CAD build for the part. Positions are in the model's coordinates, mm. A direction names the side the tool comes from. Give positions to 0.01 mm unless a question says otherwise; leave off trailing zeros. Order: outer loops, then holes, each group sorted by start corner. A loop starts at its lowest first (then second) coordinate and runs counter-clockwise, first axis right, second up.
Item 1: Wall check: L1, parallel to X at y = -5.25, z = -1.2; L2, parallel to Y at x = 15.25, z = -0.85; L3, parallel to Y at x = 32.25, z = 0.6. Give the ranges that are in metal, low to high.
Item 2: Flat gauge pins, fed straight in: P1, Ø4, axis at x = 31.46, y = -10.9, coming from the +Z side; P2, Ø2, axis at y = -8.5, z = -2, coming from the +X side; P3, Ø1.2, axis at x = 21.5, z = -1.5, coming from the -Y side; P4, Ø2.5, axis at x = 16, y = -10, coming from the -Z side. Where does each tip first touch, or does it go through?
Item 3: Two-plate mould, pull along X, no slides. Class faces 4 (the flat face through (13.37, -9.09, 0.49)), 5 (the conical face through (34.4, -13.8, 0.6)), 6 (the conical face through (6.94, -13.798, 0.618)), 7 (the flat face through (20, -13.101, -1)): released by +X, released by -X, zero draft, split by the parting line, or undercut.
Item 4: Band-saw the part on B-B on y = -8.75. Give the cut face in (x, z).
Item 5: Which spindle directions (+Z, -Z, +X, -X, +Y, -Y) get a long thin tool onto all of the face, cutting with end or side? Do faces 1 (the flat face through (7.664, -8, -1)), 2 (the flat face through (24.17, -9.09, 0.49)), 3 (the flat face through (8.9, -4.5, 0)). Say none if no direction does.
Item 6: Band-saw the part on D-D on y = -10.5. Count the separate pieces of the cut face and the enclosed holes in it, plus the area to 3 significant figures.
Item 7: Band-saw the part on A-A on z = -0.9. Give the cut face in (x, y), plus the area to 3 significant figures.
Item 8: Band-saw the part on C-C on x = 25.5. Give the cut face in (y, z), plus the area to 3 significant figures.
```python
from build123d import *

# Parameters (mm, degrees)
SKETCH_1_W          = 26
SKETCH_1_H          = 9.8
SKETCH_1_W_2        = 24
SKETCH_1_H_2        = 7.8
EXTRUDE_1_DEPTH     = 2.5
EXTRUDE_2_DEPTH     = 1
EXTRUDE_2_TAPER     = 25
CUT_EXTRUDE_1_REACH = 3
SKETCH_3_R          = 1.2


with BuildPart() as part:
    # 草图1 → 凸台-拉伸1 (new body)
    with BuildSketch(Plane.XY):
        with Locations((20.66383505, -8.200793938)):
            Rectangle(SKETCH_1_W, SKETCH_1_H)
        with Locations((20.66383505, -8.200793938)):
            Rectangle(SKETCH_1_W_2, SKETCH_1_H_2, mode=Mode.SUBTRACT)
    extrude(amount=-EXTRUDE_1_DEPTH)

    # 草图2 → 凸台-拉伸2 (add)
    with BuildSketch(Plane.XY):
        with BuildLine():
            Line((35.16383505, -12.600793938), (35.16383505, -3.800793938))
            ThreePointArc((35.16383505, -3.800793938), (34.578048612, -2.386580376), (33.16383505, -1.800793938))
            Line((33.16383505, -1.800793938), (8.16383505, -1.800793938))
            ThreePointArc((8.16383505, -1.800793938), (6.749621488, -2.386580376), (6.16383505, -3.800793938))
            Line((6.16383505, -3.800793938), (6.16383505, -12.600793938))
            ThreePointArc((6.16383505, -12.600793938), (6.749621488, -14.015007501), (8.16383505, -14.600793938))
            Line((8.16383505, -14.600793938), (33.16383505, -14.600793938))
            ThreePointArc((33.16383505, -14.600793938), (34.578048612, -14.015007501), (35.16383505, -12.600793938))
        make_face()
    extrude(amount=EXTRUDE_2_DEPTH, taper=EXTRUDE_2_TAPER)

    # 草图3 → 切除-拉伸1 (cut, up to next)
    with BuildSketch(Plane(origin=(0, 0, 0), x_dir=(-1, 0, 0), z_dir=(0, 0, -1)), mode=Mode.PRIVATE) as cut_extrude_1_sk1:
        with Locations((-31.46383505, -10.900793938)):
            Circle(SKETCH_3_R)
    cut_extrude_1_tool1 = extrude(cut_extrude_1_sk1.sketch, amount=-CUT_EXTRUDE_1_REACH, mode=Mode.PRIVATE) & part.part
    add(cut_extrude_1_tool1.solids().sort_by_distance((31.463835, -10.900794, 0))[0], mode=Mode.SUBTRACT)
    # 草图3 → 切除-拉伸1 (cut, up to next)
    with BuildSketch(Plane(origin=(0, 0, 0), x_dir=(-1, 0, 0), z_dir=(0, 0, -1)), mode=Mode.PRIVATE) as cut_extrude_1_sk2:
        with Locations((-9.86383505, -5.500793938)):
            Circle(SKETCH_3_R)
    cut_extrude_1_tool2 = extrude(cut_extrude_1_sk2.sketch, amount=-CUT_EXTRUDE_1_REACH, mode=Mode.PRIVATE) & part.part
    add(cut_extrude_1_tool2.solids().sort_by_distance((9.863835, -5.500794, 0))[0], mode=Mode.SUBTRACT)
    # 草图3 → 切除-拉伸1 (cut, up to next)
    with BuildSketch(Plane(origin=(0, 0, 0), x_dir=(-1, 0, 0), z_dir=(0, 0, -1)), mode=Mode.PRIVATE) as cut_extrude_1_sk3:
        with BuildLine():
            Line((-30.615306913, -4.652265801), (-25.215306913, -10.052265801))
            ThreePointArc((-25.215306913, -10.052265801), (-25.215306913, -11.749322076), (-26.912363188, -11.749322076))
            Line((-26.912363188, -11.749322076), (-32.312363188, -6.349322076))
            ThreePointArc((-32.312363188, -6.349322076), (-32.312363188, -4.652265801), (-30.615306913, -4.652265801))
        make_face()
    cut_extrude_1_tool3 = extrude(cut_extrude_1_sk3.sketch, amount=-CUT_EXTRUDE_1_REACH, mode=Mode.PRIVATE) & part.part
    add(cut_extrude_1_tool3.solids().sort_by_distance((28.763835, -8.200794, 0))[0], mode=Mode.SUBTRACT)
    # 草图3 → 切除-拉伸1 (cut, up to next)
    with BuildSketch(Plane(origin=(0, 0, 0), x_dir=(-1, 0, 0), z_dir=(0, 0, -1)), mode=Mode.PRIVATE) as cut_extrude_1_sk4:
        with BuildLine():
            Line((-25.215306913, -4.652265801), (-19.815306913, -10.052265801))
            ThreePointArc((-19.815306913, -10.052265801), (-19.815306913, -11.749322076), (-21.512363188, -11.749322076))
            Line((-21.512363188, -11.749322076), (-26.912363188, -6.349322076))
            ThreePointArc((-26.912363188, -6.349322076), (-26.912363188, -4.652265801), (-25.215306913, -4.652265801))
        make_face()
    cut_extrude_1_tool4 = extrude(cut_extrude_1_sk4.sketch, amount=-CUT_EXTRUDE_1_REACH, mode=Mode.PRIVATE) & part.part
    add(cut_extrude_1_tool4.solids().sort_by_distance((23.363835, -8.200794, 0))[0], mode=Mode.SUBTRACT)
    # 草图3 → 切除-拉伸1 (cut, up to next)
    with BuildSketch(Plane(origin=(0, 0, 0), x_dir=(-1, 0, 0), z_dir=(0, 0, -1)), mode=Mode.PRIVATE) as cut_extrude_1_sk5:
        with BuildLine():
            Line((-19.815306913, -4.652265801), (-14.415306913, -10.052265801))
            ThreePointArc((-14.415306913, -10.052265801), (-14.415306913, -11.749322076), (-16.112363188, -11.749322076))
            Line((-16.112363188, -11.749322076), (-21.512363188, -6.349322076))
            ThreePointArc((-21.512363188, -6.349322076), (-21.512363188, -4.652265801), (-19.815306913, -4.652265801))
        make_face()
    cut_extrude_1_tool5 = extrude(cut_extrude_1_sk5.sketch, amount=-CUT_EXTRUDE_1_REACH, mode=Mode.PRIVATE) & part.part
    add(cut_extrude_1_tool5.solids().sort_by_distance((17.963835, -8.200794, 0))[0], mode=Mode.SUBTRACT)
    # 草图3 → 切除-拉伸1 (cut, up to next)
    with BuildSketch(Plane(origin=(0, 0, 0), x_dir=(-1, 0, 0), z_dir=(0, 0, -1)), mode=Mode.PRIVATE) as cut_extrude_1_sk6:
        with BuildLine():
            Line((-14.415306913, -4.652265801), (-9.015306913, -10.052265801))
            ThreePointArc((-9.015306913, -10.052265801), (-9.015306913, -11.749322076), (-10.712363188, -11.749322076))
            Line((-10.712363188, -11.749322076), (-16.112363188, -6.349322076))
            ThreePointArc((-16.112363188, -6.349322076), (-16.112363188, -4.652265801), (-14.415306913, -4.652265801))
        make_face()
    cut_extrude_1_tool6 = extrude(cut_extrude_1_sk6.sketch, amount=-CUT_EXTRUDE_1_REACH, mode=Mode.PRIVATE) & part.part
    add(cut_extrude_1_tool6.solids().sort_by_distance((12.563835, -8.200794, 0))[0], mode=Mode.SUBTRACT)


solid = part.part
```
The answers:
1. L1: x = 7.66 to 8.66, 32.66 to 33.66
1. L2: y = -13.1 to -12.1, -4.3 to -3.3
1. L3: y = -14.32 to -11.81, -9.99 to -6.41, -4.59 to -2.08
2. P1: stops at z = 1
2. P2: stops at x = 33.66
2. P3: stops at y = -13.1
2. P4: stops at z = 0
3. face 4: undercut
3. face 5: released by +X
3. face 6: released by -X
3. face 7: zero draft
4. outline: (6.16, 0) - (7.66, 0) - (7.66, -2.5) - (8.66, -2.5) - (8.66, 0) - (10.32, 0) - (10.32, 1) - (6.63, 1) - close; (13.71, 0) - (15.72, 0) - (15.72, 1) - (13.71, 1) - close; (19.11, 0) - (21.12, 0) - (21.12, 1) - (19.11, 1) - close; (24.51, 0) - (26.52, 0) - (26.52, 1) - (24.51, 1) - close; (29.91, 0) - (32.66, 0) - (32.66, -2.5) - (33.66, -2.5) - (33.66, 0) - (35.16, 0) - (34.7, 1) - (29.91, 1) - close
5. face 1: -Z, -X, +Y, -Y
5. face 2: +Z, -Z
5. face 3: -Z
6. separate pieces: 6
6. enclosed holes: 0
6. area: 18.4 mm2
7. outline: (7.66, -13.1) - (33.66, -13.1) - (33.66, -3.3) - (7.66, -3.3) - close; hole (8.66, -12.1) - (32.66, -12.1) - (32.66, -4.3) - (8.66, -4.3) - close
7. area: 67.6 mm2
8. outline: (-14.6, 0) - (-13.1, 0) - (-13.1, -2.5) - (-12.1, -2.5) - (-12.1, 0) - (-11.96, 0) - (-11.96, 1) - (-14.13, 1) - close; (-9.77, 0) - (-7.76, 0) - (-7.76, 1) - (-9.77, 1) - close; (-4.44, 0) - (-4.3, 0) - (-4.3, -2.5) - (-3.3, -2.5) - (-3.3, 0) - (-1.8, 0) - (-2.27, 1) - (-4.44, 1) - close
8. area: 11.8 mm2
